The listing builds one solid part. Answer for the finished solid, in the listing's coordinates (mm). Give positions to 0.01 mm unless a question says otherwise; leave off trailing zeros. Write each loop counter-clockwise with the first axis right and the second up, starting at its lowest first coordinate (ties: lowest second). Pieces come first, ordered by that corner, then holes. Notation, with made-up numbers: (-23, 83.25) - (6, 83.25) arc R27 ccw to (6, 122.25) - close; hole circle Ø5 at (-34.5, 28). An arc over 180 degrees is marked (long way). Write each question's results on one line, items separated by ' | '. Start each with the question number.
Q1. Flat-ended cylindrical pins translate along their axes: pin 1 Ø1.8 at (x, y) = (45, -63) entering from -Z; pin 2 Ø1.6 at (x, z) = (-51, 0.5) entering from +Y; pin 3 Ø2 at (x, z) = (17.5, 1.5) entering from -Y; pin 4 Ø1.6 at (y, z) = (-62, 1) entering from -X. Find the tip coordinate at first contact, or state that the pin passes through.
Q2. Section C-C (x = 51.5) is taken. Determine the outline of the cut face in (y, z).
Q3. Section D-D (x = -9) is taken. Determine the outline of the cut face in (y, z), plus the area to 3 significant figures.
Q4. Find the intervals of material crossed by probe 1 along X at (y, z) = (42, -0.9); probe 2 along Y at (x, z) = (45, 0.65); probe 3 along Y at (x, z) = (45, -2.05), in increasing order.
Q5. Section B-B (x = -45) is taken. Determine the outline of the cut face in (y, z), plus the area to 3 significant figures.
Q6. Section A-A (z = 0.25) is taken. Determine the outline of the cut face in (x, y).
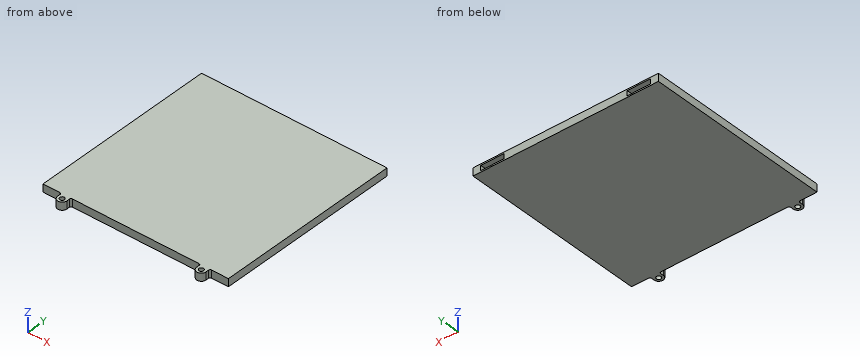
```python
from build123d import *

# Parameters (mm, degrees)
SKETCH1_W            = 120
SKETCH1_H            = 120
BOSS_EXTRUDE1_DEPTH  = 2.5
SKETCH4_W            = 15.2
SKETCH4_H            = 3.2
CUT_EXTRUDE1_DEPTH   = 20
SKETCH6_R            = 1.5
BOSS_EXTRUDE2_DEPTH  = 5
FILLET1_R            = 1
FILLET1_OF_MIRROR1_R = 1


with BuildPart() as part:
    # Sketch1 → Boss-Extrude1 (new body, symmetric)
    with BuildSketch(Plane.XY):
        Rectangle(SKETCH1_W, SKETCH1_H)
    extrude(amount=BOSS_EXTRUDE1_DEPTH, both=True)

    # Sketch4 → Cut-Extrude1 (cut)
    with BuildSketch(Plane(origin=(0, 60, 0), x_dir=(1, 0, 0), z_dir=(0, 1, 0))):
        with Locations((-47.4, 0)):
            Rectangle(SKETCH4_W, SKETCH4_H)
        with Locations((47.4, 0)):
            Rectangle(SKETCH4_W, SKETCH4_H)
    extrude(amount=-CUT_EXTRUDE1_DEPTH, mode=Mode.SUBTRACT)

    # Sketch6 → Boss-Extrude2 (add)
    with BuildSketch(Plane.XY.offset(2.5)):
        with BuildLine():
            Line((42, -60), (48, -60))
            Line((48, -60), (48, -63))
            ThreePointArc((48, -63), (45, -66), (42, -63))
            Line((42, -63), (42, -60))
        make_face()
        with Locations((45, -63)):
            Circle(SKETCH6_R, mode=Mode.SUBTRACT)
    boss_extrude2 = extrude(amount=-BOSS_EXTRUDE2_DEPTH)

    # Fillet1
    fillet1_edges = [part.edges().sort_by_distance(p)[0] for p in [
        (42, -60, 0),
        (48, -60, 0),
    ]]
    fillet(fillet1_edges, radius=FILLET1_R)

    # Mirror1: Boss-Extrude2 across plane
    add(boss_extrude2.mirror(Plane(origin=(0, 0, 0), x_dir=(0, 0, 1), z_dir=(1, 0, 0))))

    # Fillet1 of Mirror1
    fillet1_of_mirror1_edges = [part.edges().sort_by_distance(p)[0] for p in [
        (-42, -60, 0),
        (-48, -60, 0),
    ]]
    fillet(fillet1_of_mirror1_edges, radius=FILLET1_OF_MIRROR1_R)


solid = part.part
```
Answers below:
1) pin 1: passes through | pin 2: stops at y = 40 | pin 3: stops at y = -60 | pin 4: stops at x = -48
2) outline: (-60, -2.5) - (60, -2.5) - (60, -1.6) - (40, -1.6) - (40, 1.6) - (60, 1.6) - (60, 2.5) - (-60, 2.5) - close
3) outline: (-60, -2.5) - (60, -2.5) - (60, 2.5) - (-60, 2.5) - close | area: 600 mm2
4) probe 1: x = -60 to -55, -39.8 to 39.8, 55 to 60 | probe 2: y = -66 to -64.5, -61.5 to 40 | probe 3: y = -66 to -64.5, -61.5 to 60
5) outline: (-66, -2.5) - (-64.5, -2.5) - (-64.5, 2.5) - (-66, 2.5) - close; (-61.5, -2.5) - (60, -2.5) - (60, -1.6) - (40, -1.6) - (40, 1.6) - (60, 1.6) - (60, 2.5) - (-61.5, 2.5) - close | area: 551 mm2
6) outline: (-60, -60) - (-49, -60) arc R1 cw to (-48, -61) - (-48, -63) arc R3 ccw to (-42, -63) - (-42, -61) arc R1 cw to (-41, -60) - (41, -60) arc R1 cw to (42, -61) - (42, -63) arc R3 ccw to (48, -63) - (48, -61) arc R1 cw to (49, -60) - (60, -60) - (60, 60) - (55, 60) - (55, 40) - (39.8, 40) - (39.8, 60) - (-39.8, 60) - (-39.8, 40) - (-55, 40) - (-55, 60) - (-60, 60) - close; hole circle Ø3 at (-45, -63); hole circle Ø3 at (45, -63)
